CAD build for the part. Positions are in the model's coordinates, mm. Face numbers are marked on the shaded views. Coordinates: 2 decimals unless noted, no trailing zeros. Order: outer loops, then holes, each group sorted by start corner. A loop starts at its lowest first (then second) coordinate and runs counter-clockwise, first axis right, second up. Notation, with made-up numbers: (76.25, -37.75) - (132.25, -37.75) arc R15 ccw to (132.25, -31.75) - close; hole circle Ø11 at (-9.5, 84). An arc over 180 degrees is marked (long way). Use one line per item in the form item = value.
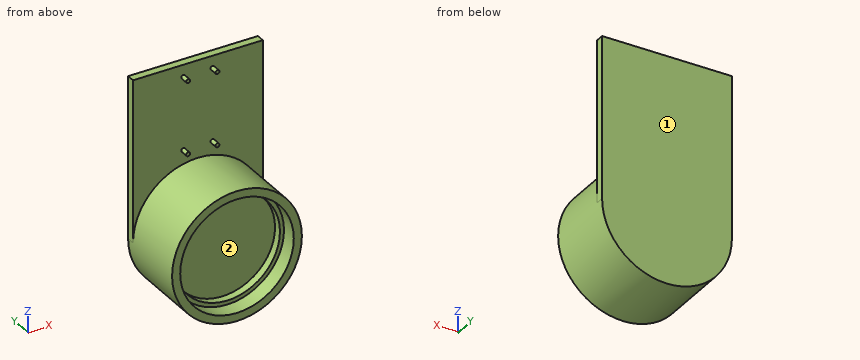
```python
from build123d import *

# Parameters (mm, degrees)
F0_R     = 1.25
F1_DEPTH = 5
F2_DEPTH = 45
F3_DEPTH = 35
F4_DEPTH = 30
F5_DEPTH = 10


with BuildPart() as f1:
    # F0 (on Front) → F1 (new body)
    with BuildSketch(Plane.XZ):
        with BuildLine():
            Line((0.7988151149, 94.5963411382), (-79.2011848851, 94.5963411382))
            Line((-79.2011848851, 94.5963411382), (-79.2011848851, -5.4036588618))
            ThreePointArc((-79.2011848851, -5.4036588618), (-39.2011848851, 34.5963411382), (0.7988151149, -5.4036588618))
            Line((0.7988151149, -5.4036588618), (0.7988151149, 94.5963411382))
        make_face()
        with Locations((-48.2011848851, 42.0963411382)):
            Circle(F0_R, mode=Mode.SUBTRACT)
        with Locations((-48.2011848851, 87.0963411382)):
            Circle(F0_R, mode=Mode.SUBTRACT)
        with Locations((-30.2011848851, 42.0963411382)):
            Circle(F0_R, mode=Mode.SUBTRACT)
        with Locations((-30.2011848851, 87.0963411382)):
            Circle(F0_R, mode=Mode.SUBTRACT)
    extrude(amount=F1_DEPTH)

    # F0 (on Front) → F2 (join)
    with BuildSketch(Plane.XZ):
        with BuildLine():
            Line((-74.2011848851, -5.4036588618), (-79.2011848851, -5.4036588618))
            ThreePointArc((-79.2011848851, -5.4036588618), (-39.2011848851, -45.4036588618), (0.7988151149, -5.4036588618))
            Line((0.7988151149, -5.4036588618), (-4.2011848851, -5.4036588618))
            ThreePointArc((-4.2011848851, -5.4036588618), (-39.2011848851, -40.4036588618), (-74.2011848851, -5.4036588618))
        make_face()
        with BuildLine():
            ThreePointArc((0.7988151149, -5.4036588618), (-39.2011848851, 34.5963411382), (-79.2011848851, -5.4036588618))
            Line((-79.2011848851, -5.4036588618), (-74.2011848851, -5.4036588618))
            ThreePointArc((-74.2011848851, -5.4036588618), (-39.2011848851, 29.5963411382), (-4.2011848851, -5.4036588618))
            Line((-4.2011848851, -5.4036588618), (0.7988151149, -5.4036588618))
        make_face()
    extrude(amount=F2_DEPTH)

    # F0 (on Front) → F3 (join)
    with BuildSketch(Plane.XZ):
        with BuildLine():
            ThreePointArc((-4.2011848851, -5.4036588618), (-39.2011848851, 29.5963411382), (-74.2011848851, -5.4036588618))
            Line((-74.2011848851, -5.4036588618), (-71.7011848851, -5.4036588618))
            ThreePointArc((-71.7011848851, -5.4036588618), (-39.2011848851, 27.0963411382), (-6.7011848851, -5.4036588618))
            Line((-6.7011848851, -5.4036588618), (-4.2011848851, -5.4036588618))
        make_face()
        with BuildLine():
            Line((-71.7011848851, -5.4036588618), (-74.2011848851, -5.4036588618))
            ThreePointArc((-74.2011848851, -5.4036588618), (-39.2011848851, -40.4036588618), (-4.2011848851, -5.4036588618))
            Line((-4.2011848851, -5.4036588618), (-6.7011848851, -5.4036588618))
            ThreePointArc((-6.7011848851, -5.4036588618), (-39.2011848851, -37.9036588618), (-71.7011848851, -5.4036588618))
        make_face()
    extrude(amount=F3_DEPTH)

    # F0 (on Front) → F4 (join)
    with BuildSketch(Plane.XZ):
        with BuildLine():
            ThreePointArc((-6.7011848851, -5.4036588618), (-39.2011848851, 27.0963411382), (-71.7011848851, -5.4036588618))
            Line((-71.7011848851, -5.4036588618), (-6.7011848851, -5.4036588618))
        make_face()
        with BuildLine():
            Line((-6.7011848851, -5.4036588618), (-71.7011848851, -5.4036588618))
            ThreePointArc((-71.7011848851, -5.4036588618), (-39.2011848851, -37.9036588618), (-6.7011848851, -5.4036588618))
        make_face()
    extrude(amount=F4_DEPTH)

    # F0 (on Front) → F5 (join)
    with BuildSketch(Plane.XZ):
        with Locations((-30.2011848851, 42.0963411382)):
            Circle(F0_R)
        with Locations((-48.2011848851, 42.0963411382)):
            Circle(F0_R)
        with Locations((-48.2011848851, 87.0963411382)):
            Circle(F0_R)
        with Locations((-30.2011848851, 87.0963411382)):
            Circle(F0_R)
    extrude(amount=F5_DEPTH)


solid = f1.part
```
Item 1: Cut at A-A, the plane y = -39.5. Write the cut outline in (x, z), plus the area to 3 significant figures.
Derived:
outline = circle Ø80 at (-39.2, -5.4); hole circle Ø70 at (-39.2, -5.4)
area = 1,180 mm²
Item 2: Cut at D-D, the plane y = -26.5. Write the cut outline in (x, z).
Derived:
outline = circle Ø80 at (-39.2, -5.4)
Item 3: Two-plate mould, pull along Z, no slides. Class the marked faces 1 and 2: +Z half, -Z half, draft (parallel to the pull), parting line (faces both ways), or undercut.
Derived:
face_1 = draft
face_2 = undercut
Item 4: Drill centre lines: line 1 (Y direction, x = -37, z = -37); line 2 (Y direction, x = -6, z = 74.5); line 3 (Z direction, x = -49, y = -39). Where is each one in solid material? Low to high. Write a range as [from, to].
Derived:
line_1 = [-30, 0]
line_2 = [-5, 0]
line_3 = [-44.18, -39], [28.2, 33.38]
Item 5: Cut at B-B, the plane z = -3. Write the cut outline in (x, y).
Derived:
outline = (-79.2, -5) - (-79.13, -5) - (-79.13, -45) - (-74.12, -45) - (-74.12, -35) - (-71.61, -35) - (-71.61, -30) - (-6.79, -30) - (-6.79, -35) - (-4.28, -35) - (-4.28, -45) - (0.73, -45) - (0.73, -5) - (0.8, -5) - (0.8, 0) - (-79.2, 0) - close
Item 6: Cut at C-C, the plane x = -58.5. Write the cut outline in (y, z).
Derived:
outline = (-45, -40.44) - (0, -40.44) - (0, 94.6) - (-5, 94.6) - (-5, 29.63) - (-45, 29.63) - (-45, 23.79) - (-35, 23.79) - (-35, 20.75) - (-30, 20.75) - (-30, -31.55) - (-35, -31.55) - (-35, -34.6) - (-45, -34.6) - close
Item 7: Drop flat-ended pins along their axis: pin 1 (0.8 mm diameter, centred on x = -48, z = 86.5, fed in from -Y); pin 2 (24 mm diameter, centred on x = -52.5, z = 69, fed in from -Y); pin 3 (5 mm diameter, centred on x = -61.5, y = -9, fed in from -Z). Give the stop position or say it passes through.
Derived:
pin_1 = -10
pin_2 = -5
pin_3 = -40.16
